The figure shows three views and two pictorial views of one solid part (mm, origin at its lowest corner). Answer the questions. Coordinates: 2 decimals unless noted, no trailing zeros. Loops run counter-clockwise (first coordinate to the right, second up) from the corner with the lowest first, then second, coordinate; pieces in that order, holes last. Notation, with made-up numbers: M -34.75,13 L 7.25,13 A8 ccw 7.25,27 Z; hole C -40,-21.75 d2. An arc over 180 degrees is marked long. Return JSON: item names as keys, results as strings. Group by question number.
1. Given P1, Ø4, axis at x = 7.5, y = 49, coming from the -Z side, flat-ended and moving along its own axis, determine where the tip first touches the part or whether it passes through.
2. Section B-B (z = 5.5) is taken. Write down the section's boundary in (x, y).
3. Section C-C (y = 32) is taken. Write down the section's boundary in (x, z), then the cut area to 3 significant figures.
4. Straight lines are drawn through the part: L1, parallel to X at y = 54, z = 7.25; L2, parallel to Y at x = 8.5, z = 8.5. For each, find the intervals that lie inside material, in ascending order. Write a range as from..to.
5. The mould has two halves that part along Y. Classify the marked faces 1, 2, 3 and 4: pulls with the +Y half, pulls with the -Y half, needs draft (parallel to the pull), parting line crosses it, or undercut.
6. Section A-A (x = 7.5) is taken. Write down the section's boundary in (y, z), then the cut area to 3 significant figures.
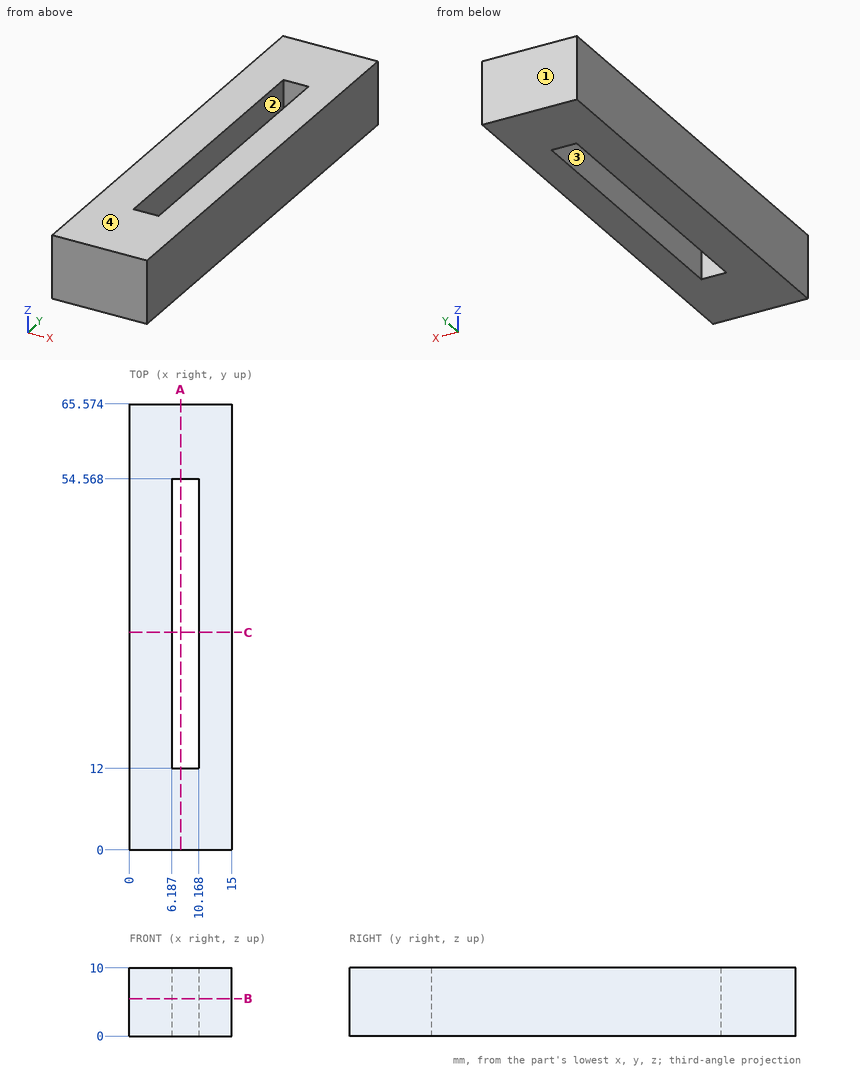
Worked out:
{
 "1": {"P1": "z = 0"},
 "2": {"outline": "M 0,0 L 15,0 L 15,65.57 L 0,65.57 Z; hole M 6.19,12 L 10.17,12 L 10.17,54.57 L 6.19,54.57 Z"},
 "3": {"outline": "M 0,0 L 6.19,0 L 6.19,10 L 0,10 Z; M 10.17,0 L 15,0 L 15,10 L 10.17,10 Z", "area": "110 mm^2"},
 "4": {"L1": "0..6.19, 10.17..15", "L2": "0..12, 54.57..65.57"},
 "5": {"face 1": "pulls with the +Y half", "face 2": "undercut", "face 3": "undercut", "face 4": "needs draft"},
 "6": {"outline": "M 0,0 L 12,0 L 12,10 L 0,10 Z; M 54.57,0 L 65.57,0 L 65.57,10 L 54.57,10 Z", "area": "230 mm^2"}
}
